Study the drawing (mm; zero at the part's minimum x, y, z) and answer. A direction names the side the tool comes from. Give positions to 0.01 mm unless a question says otherwise; leave off trailing zeros. Loops run counter-clockwise (first coordinate to the right, second up) from the corner with the lowest first, then second, coordinate; pieces in that order, holes last. Notation, with made-up numbers: (25.5, -10.75) - (73.5, -10.75) arc R25 ccw to (73.5, 1.25) - close; hole circle Ø2 at (85.25, 46). An arc over 180 degrees is marked (long way). Write item = value, one per line. Start each with the question number.
1) The mould has two halves that part along X. Classify the marked faces 3, 4 and 5: +X half, -X half, draft (parallel to the pull), parting line (faces both ways), or undercut.
2) The part is cut by section C-C on y = 108.5. Write down the section's boundary in (x, z), plus the area to 3 significant figures.
3) The part is cut by section A-A on x = 16.2. Write down the section's boundary in (y, z), plus the area to 3 significant figures.
4) Which of the six approach directions +Z, -Z, +X, -X, +Y, -Y give full straight-line access (tool end or side, diameter ignored) to the marked faces 1 and 2?
5) Consider probe 1 along X at (y, z) = (44.5, 1.1); probe 2 along X at (y, z) = (107, 11.25); probe 3 along Y at (x, z) = (36.2, 2.2). Determine where each line is inside the solid, lowest interval first.
6) The part is cut by section B-B on z = 18.25. Write down the section's boundary in (x, y).
7) The part is cut by section D-D on y = 25. Write down the section's boundary in (x, z), plus the area to 3 significant figures.
8) A flat-ended cylindrical pin translates along its axis: P1, Ø8, axis at x = 45, y = 119, coming from the +Z side. Find the tip coordinate at first contact, or state that the pin passes through.
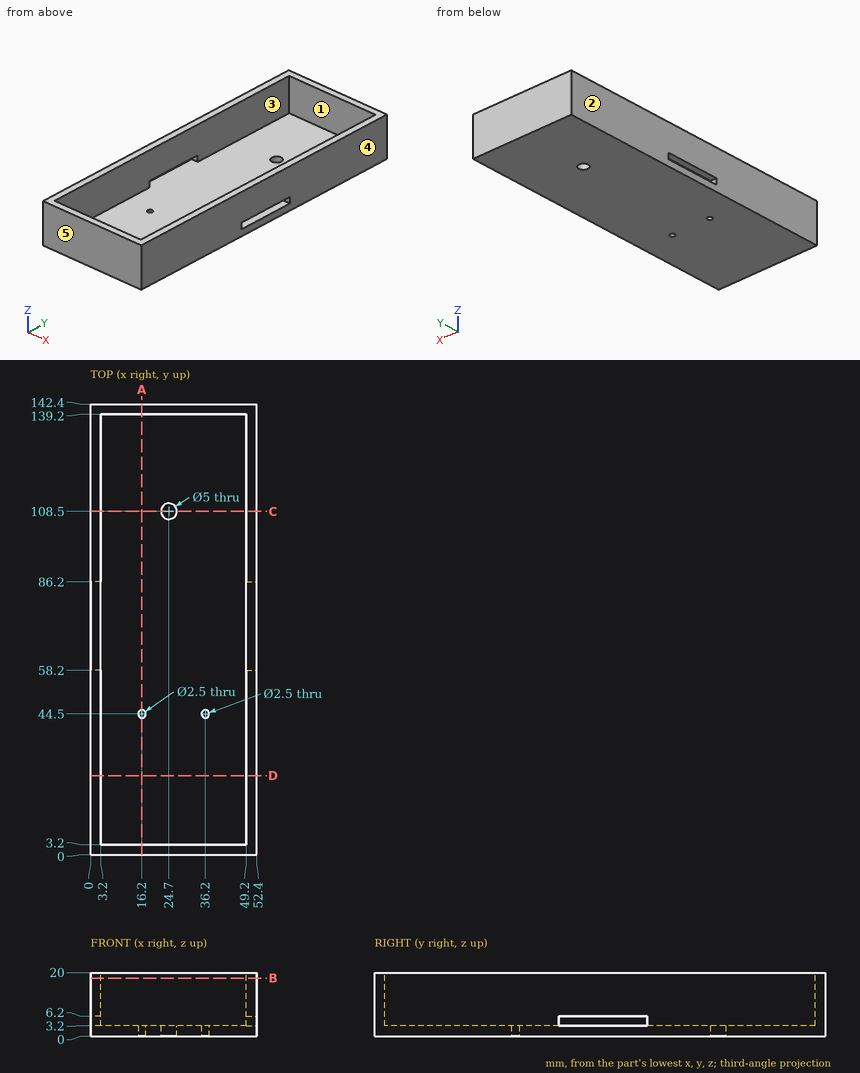
Answer below:
q1.face_3 = undercut
q1.face_4 = +X half
q1.face_5 = draft
q2.outline = (0, 0) - (22.2, 0) - (22.2, 3.2) - (3.2, 3.2) - (3.2, 20) - (0, 20) - close; (27.2, 0) - (52.4, 0) - (52.4, 20) - (49.2, 20) - (49.2, 3.2) - (27.2, 3.2) - close
q2.area = 259 mm2
q3.outline = (0, 0) - (43.25, 0) - (43.25, 3.2) - (3.2, 3.2) - (3.2, 20) - (0, 20) - close; (45.75, 0) - (142.4, 0) - (142.4, 20) - (139.2, 20) - (139.2, 3.2) - (45.75, 3.2) - close
q3.area = 555 mm2
q4.face_1 = +Z
q4.face_2 = +Z, -Z, -X, +Y, -Y
q5.probe_1 = 0 to 14.95, 17.45 to 34.95, 37.45 to 52.4
q5.probe_2 = 0 to 3.2, 49.2 to 52.4
q5.probe_3 = 0 to 43.25, 45.75 to 142.4
q6.outline = (0, 0) - (52.4, 0) - (52.4, 142.4) - (0, 142.4) - close; hole (3.2, 3.2) - (49.2, 3.2) - (49.2, 139.2) - (3.2, 139.2) - close
q7.outline = (0, 0) - (52.4, 0) - (52.4, 20) - (49.2, 20) - (49.2, 3.2) - (3.2, 3.2) - (3.2, 20) - (0, 20) - close
q7.area = 275 mm2
q8.P1 = 3.2
